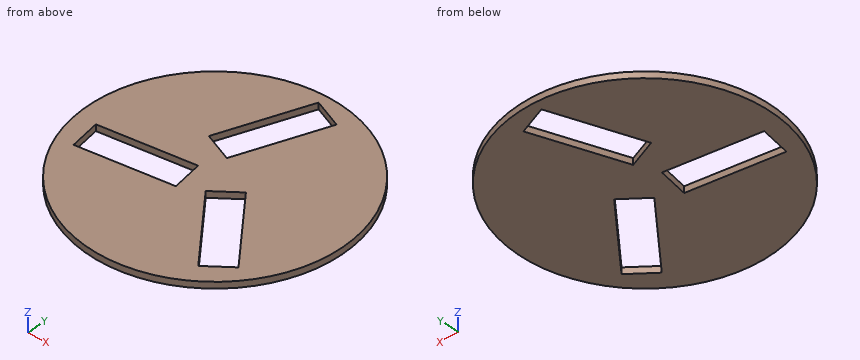
```python
from build123d import *

# Parameters (mm, degrees)
F0_R     = 94
F2_DEPTH = 4.7
F5_DEPTH = 4.8


with BuildPart() as f2:
    # F0 (on Top) → F2 (new body)
    with BuildSketch(Plane.XY):
        with Locations((0, 3.286633)):
            Circle(F0_R)
    extrude(amount=-F2_DEPTH)

    # F1 (on Top) + F3 (on Top) + F4 (on Top) → F5 (cut)
    with BuildSketch(Plane.XY):
        Polygon((21.988586, 4.168563), (4.870629, -9.650827), (46.956953, -61.782787), (64.07491, -47.963397), align=None)
    with BuildSketch(Plane.XY):
        Polygon((-26.944155, 27.743882), (-6.417233, 19.828992), (17.687206, 82.342798), (-2.839715, 90.257689), align=None)
    with BuildSketch(Plane.XY):
        Polygon((-10.029213, -17.480458), (-13.438177, 4.253823), (-79.628941, -6.128023), (-76.219977, -27.862304), align=None)
    extrude(amount=-F5_DEPTH, mode=Mode.SUBTRACT)


solid = f2.part
```
Model file for the job. Use its own axes, mm. Give positions to 0.01 mm unless a question says otherwise; leave off trailing zeros. Write each loop counter-clockwise with the first axis right and the second up, starting at its lowest first coordinate (ties: lowest second). Pieces come first, ordered by that corner, then holes. Notation, with made-up numbers: (23, 69.25) -> (34, 69.25) arc R18 cw to (34, 96.25) -> close; hole circle Ø10 at (14.25, 17). An arc over 180 degrees is marked (long way). Use CSV: the item, a comma, the result in double quotes. Start each with the question number.
1) Cut at A-A on y = 65.5. List the corners of the cut face in (x, z).
2) Cut at D-D on x = -82. List the corners of the cut face in (y, z), plus the area to 3 significant figures.
3) Pin check, flat tips, straight feed: P1, Ø1.5, axis at x = 4.5, z = -1.5, coming from the +Y side; P2, Ø2, axis at y = 52, z = -3, coming from the -X side. Stop position of each tip, or through.
4) Cut at B-B on z = -2.2. List the corners of the cut face in (x, y), plus the area to 3 significant figures.
5) Cut at C-C on x = 0. List the corners of the cut face in (y, z), plus the area to 3 significant figures.
6) Drill centre lines: L1, parallel to Y at x = -64.5, z = -4; L2, parallel to Y at x = -66.5, z = -4.2; L3, parallel to X at y = 40, z = -3.3. Where is each one in solid material? Low to high.
Final values:
1,outline,"(-70.47, -4.7) -> (-12.39, -4.7) -> (-12.39, 0) -> (-70.47, 0) -> close; (11.19, -4.7) -> (70.47, -4.7) -> (70.47, 0) -> (11.19, 0) -> close"
2,outline,"(-42.67, -4.7) -> (49.24, -4.7) -> (49.24, 0) -> (-42.67, 0) -> close"
2,area,"432 mm2"
3,P1,"stops at y = 97.21"
3,P2,"stops at x = -80.99"
4,outline,"circle Ø188 at (0, 3.29); hole (-79.63, -6.13) -> (-76.22, -27.86) -> (-10.03, -17.48) -> (-13.44, 4.25) -> close; hole (-26.94, 27.74) -> (-6.42, 19.83) -> (17.69, 82.34) -> (-2.84, 90.26) -> close; hole (4.87, -9.65) -> (46.96, -61.78) -> (64.07, -47.96) -> (21.99, 4.17) -> close"
4,area,"23,300 mm2"
5,outline,"(-90.71, -4.7) -> (36.47, -4.7) -> (36.47, 0) -> (-90.71, 0) -> close; (89.16, -4.7) -> (97.29, -4.7) -> (97.29, 0) -> (89.16, 0) -> close"
5,area,"636 mm2"
6,L1,"y = -65.09 to -26.02, -3.76 to 71.67"
6,L2,"y = -63.15 to -26.34, -4.07 to 69.72"
6,L3,"x = -86.53 to -22.22, 1.36 to 86.53"
